Source: CAD feature listing. Evaluate the final solid. Frame: model axes, mm. Face numbers are marked on the shaded views. A direction names the side the tool comes from. Coordinates: 2 decimals unless noted, no trailing zeros. Write each loop counter-clockwise with the first axis right and the second up, starting at its lowest first coordinate (ties: lowest second). Pieces come first, ordered by that corner, then holes. Notation, with made-up numbers: (54.25, -23.5) - (112.25, -23.5) arc R29 cw to (112.25, 3.5) - close; hole circle Ø7 at (33, -8). An arc over 180 degrees is marked (long way). One line per item, written item: value.
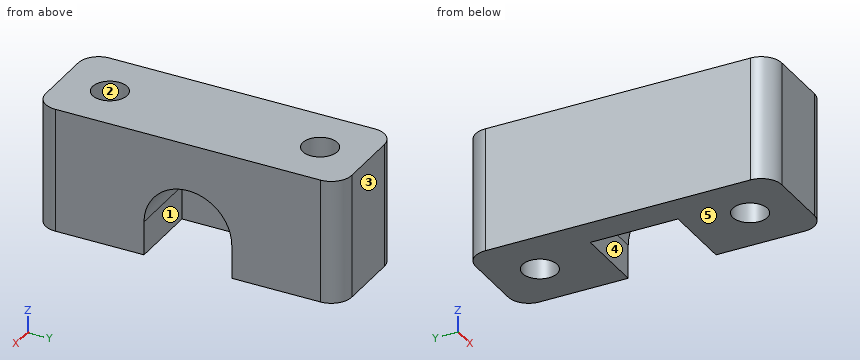
from build123d import *

# Parameters (mm, degrees)
SKETCH1_W           = 12.2
SKETCH1_H           = 30
BOSS_EXTRUDE1_DEPTH = 5
SKETCH5_R           = 4.3
CUT_EXTRUDE2_DEPTH  = 7
SKETCH3_R           = 1.7
CUT_EXTRUDE1_DEPTH  = 20.970978944
FILLET1_R           = 2
FILLET2_R           = 0.1
CUT_EXTRUDE3_DEPTH  = 7


with BuildPart() as part:
    # Sketch1 → Boss-Extrude1 (new, symmetric)
    with BuildSketch(Plane(origin=(0, 0, 0), x_dir=(0, 0, -1), z_dir=(1, 0, 0))):
        Rectangle(SKETCH1_W, SKETCH1_H)
    extrude(amount=BOSS_EXTRUDE1_DEPTH, both=True)

    # Sketch5 → Cut-Extrude2 (cut)
    with BuildSketch(Plane(origin=(5, 0, 0), x_dir=(0, 0, -1), z_dir=(1, 0, 0))):
        with Locations((2.8, 0)):
            Circle(SKETCH5_R)
    extrude(amount=-CUT_EXTRUDE2_DEPTH, mode=Mode.SUBTRACT)

    # Sketch3 → Cut-Extrude1 (cut, through all)
    with BuildSketch(Plane.XY.offset(6.1)):
        with Locations((0, 10.3)):
            Circle(SKETCH3_R)
    cut_extrude1 = extrude(amount=-CUT_EXTRUDE1_DEPTH, mode=Mode.SUBTRACT)

    # Mirror1: Cut-Extrude1 across plane
    add(cut_extrude1.mirror(Plane.ZX), mode=Mode.SUBTRACT)

    # Fillet1
    fillet1_edges = [part.edges().sort_by_distance(p)[0] for p in [
        (5, -15, 0),
        (-5, -15, 0),
        (-5, 15, 0),
        (5, 15, 0),
    ]]
    fillet(fillet1_edges, radius=FILLET1_R)

    # Fillet2
    fillet2_edges = [part.edges().sort_by_distance(p)[0] for p in [
        (1.5, -2.75680975, -6.1),
        (1.5, 2.75680975, -6.1),
    ]]
    fillet(fillet2_edges, radius=FILLET2_R)

    # Sketch6 → Cut-Extrude3 (cut)
    with BuildSketch(Plane(origin=(5, 0, 0), x_dir=(0, 0, -1), z_dir=(1, 0, 0))):
        with BuildLine():
            Line((2.8, 4.3), (6.1, 4.3))
            ThreePointArc((6.1, 4.3), (10.4, 0), (6.1, -4.3))
            Line((6.1, -4.3), (2.8, -4.3))
            ThreePointArc((2.8, -4.3), (-1.5, 0), (2.8, 4.3))
        make_face()
    extrude(amount=-CUT_EXTRUDE3_DEPTH, mode=Mode.SUBTRACT)


solid = part.part
1) Section query D-D on x = 0. Output: boundary loops of the cut face in (y, z).
Values found:
outline: (-15, -6.1) - (-12, -6.1) - (-12, 6.1) - (-15, 6.1) - close; (-8.6, -6.1) - (-4.3, -6.1) - (-4.3, -2.8) arc R4.3 cw to (4.3, -2.8) - (4.3, -6.1) - (8.6, -6.1) - (8.6, 6.1) - (-8.6, 6.1) - close; (12, -6.1) - (15, -6.1) - (15, 6.1) - (12, 6.1) - close
2) Draft query along Y for the marked faces 3, 4 and 5. Return one class per face: released by +Y, released by -Y, zero draft, split by the parting line, or undercut.
Values found:
face 3: released by +Y
face 4: undercut
face 5: zero draft
3) Section query C-C on z = 2.5. Output: boundary loops of the cut face in (x, y), then the cut area to 3 significant figures.
Values found:
outline: (-5, -13) arc R2 ccw to (-3, -15) - (3, -15) arc R2 ccw to (5, -13) - (5, 13) arc R2 ccw to (3, 15) - (-3, 15) arc R2 ccw to (-5, 13) - close; hole circle Ø3.4 at (0, -10.3); hole circle Ø3.4 at (0, 10.3)
area: 278 mm2
4) Material intervals for line 1 (Y direction, x = 0, z = 2); line 2 (Y direction, x = 0, z = -3); line 3 (Y direction, x = 0, z = 1), sorted ascending.
Values found:
line 1: -15 to -12, -8.6 to 8.6, 12 to 15
line 2: -15 to -12, -8.6 to -4.3, 4.3 to 8.6, 12 to 15
line 3: -15 to -12, -8.6 to -2.01, 2.01 to 8.6, 12 to 15
5) Reachability of the marked faces 1 and 2 from +Z, -Z, +X, -X, +Y, -Y: full face, straight path, thin tool, end or side. Return the list, or none.
Values found:
face 1: -Z, +X
face 2: +Z, -Z
6) Section query A-A on y = 10.3. Output: boundary loops of the cut face in (x, z).
Values found:
outline: (-5, -6.1) - (-1.7, -6.1) - (-1.7, 6.1) - (-5, 6.1) - close; (1.7, -6.1) - (5, -6.1) - (5, 6.1) - (1.7, 6.1) - close
7) Section query B-B on x = 2.25. Output: boundary loops of the cut face in (y, z), then the cut area to 3 significant figures.
Values found:
outline: (-15, -6.1) - (-4.3, -6.1) - (-4.3, -2.8) arc R4.3 cw to (4.3, -2.8) - (4.3, -6.1) - (15, -6.1) - (15, 6.1) - (-15, 6.1) - close
area: 309 mm2
8) Contact query for flat-ended pins moving along their axis: P1, Ø2.5, axis at x = 0, y = 10.3, coming from the +Z side; P2, Ø2.5, axis at y = 2, z = -1.5, coming from the +X side. Output: stop coordinate, or through.
Values found:
P1: through
P2: x = -2
